Read the model definition and answer for the solid it produces. Units are mm, in the model's axes. Face numbers are marked on the shaded views. A direction names the side the tool comes from. Round coordinates to 2 decimals unless told otherwise and drop trailing zeros. Loops run counter-clockwise (first coordinate to the right, second up) from the corner with the lowest first, then second, coordinate; pieces in that order, holes last. Notation, with made-up numbers: (25.5, 24.25) -> (54.5, 24.25) arc R25 ccw to (54.5, 55.25) -> close; hole circle Ø10 at (-12.75, -29.5). An arc over 180 degrees is marked (long way). Put each result on its own line as item: value.
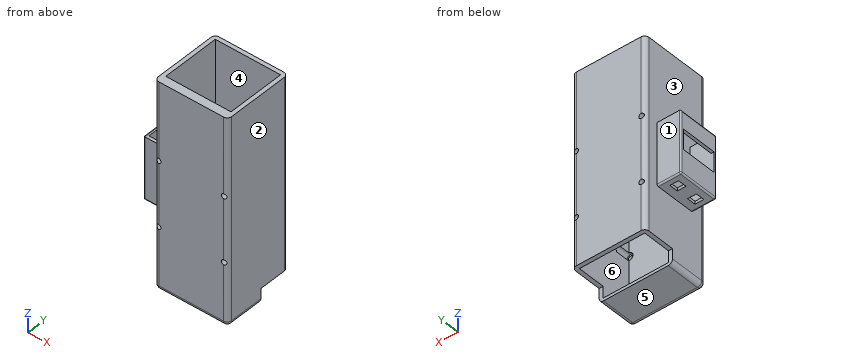
from build123d import *

# Parameters (mm, degrees)
SKETCH1_W           = 50.6
SKETCH1_H           = 45.6
SKETCH1_W_2         = 45
SKETCH1_H_2         = 40
BOSS_EXTRUDE1_DEPTH = 70
SKETCH2_W           = 50.6
SKETCH2_H           = 45.6
BOSS_EXTRUDE2_DEPTH = 2
SKETCH4_R           = 1.7
CUT_EXTRUDE1_DEPTH  = 71.5
SKETCH5_R           = 2.75
CUT_EXTRUDE2_DEPTH  = 12.5
SKETCH6_W           = 50.6
SKETCH6_H           = 4.293520681
BOSS_EXTRUDE3_DEPTH = 142
SKETCH7_R           = 1.7
CUT_EXTRUDE3_DEPTH  = 7.5
FILLET1_R           = 3
CUT_EXTRUDE4_DEPTH  = 22
BOSS_EXTRUDE4_DEPTH = 14.5
SKETCH10_W          = 43
SKETCH10_H          = 28.7
BOSS_EXTRUDE5_DEPTH = 2
SKETCH11_W          = 14
SKETCH11_H          = 24.7
CUT_EXTRUDE5_DEPTH  = 2
SKETCH12_W          = 6
SKETCH12_H          = 6
CUT_EXTRUDE6_DEPTH  = 2
FILLET2_R           = 1


with BuildPart() as part:
    # Sketch1 → Boss-Extrude1 (new, symmetric)
    with BuildSketch(Plane.XY):
        Rectangle(SKETCH1_W, SKETCH1_H)
        Rectangle(SKETCH1_W_2, SKETCH1_H_2, mode=Mode.SUBTRACT)
    extrude(amount=BOSS_EXTRUDE1_DEPTH, both=True)

    # Sketch2 → Boss-Extrude2 (add)
    with BuildSketch(Plane(origin=(0, 0, -70), x_dir=(-1, 0, 0), z_dir=(0, 0, -1))):
        Rectangle(SKETCH2_W, SKETCH2_H)
    extrude(amount=BOSS_EXTRUDE2_DEPTH)

    # Sketch4 → Cut-Extrude1 (cut)
    with BuildSketch(Plane(origin=(0, 22.8, 0), x_dir=(1, 0, 0), z_dir=(0, 1, 0))):
        with Locations(Location((-22.534370918, 28.890457594, 0), (0, 0, 270))):
            Circle(SKETCH4_R)
        with Locations(Location((22.465629082, 28.890457594, 0), (0, 0, 270))):
            Circle(SKETCH4_R)
        with Locations(Location((22.465629082, -16.109542406, 0), (0, 0, 270))):
            Circle(SKETCH4_R)
        with Locations(Location((-22.534370918, -16.109542406, 0), (0, 0, 270))):
            Circle(SKETCH4_R)
    extrude(amount=-CUT_EXTRUDE1_DEPTH, mode=Mode.SUBTRACT)

    # Sketch5 → Cut-Extrude2 (cut)
    with BuildSketch(Plane(origin=(0, -10, 0), x_dir=(1, 0, 0), z_dir=(0, 1, 0))):
        with Locations(Location((22.465629082, 28.890457594, 0), (0, 0, 270))):
            Circle(SKETCH5_R)
        with Locations(Location((22.465629082, -16.109542406, 0), (0, 0, 270))):
            Circle(SKETCH5_R)
        with Locations(Location((-22.534370918, 28.890457594, 0), (0, 0, 270))):
            Circle(SKETCH5_R)
        with Locations(Location((-22.534370918, -16.109542406, 0), (0, 0, 270))):
            Circle(SKETCH5_R)
    extrude(amount=-CUT_EXTRUDE2_DEPTH, mode=Mode.SUBTRACT)

    # Sketch6 → Boss-Extrude3 (add)
    with BuildSketch(Plane.XY.offset(70)):
        with Locations((0, -23.65323966)):
            Rectangle(SKETCH6_W, SKETCH6_H)
    extrude(amount=-BOSS_EXTRUDE3_DEPTH)

    # Sketch7 → Cut-Extrude3 (cut)
    with BuildSketch(Plane(origin=(0, -21.506479319, 0), x_dir=(1, 0, 0), z_dir=(0, 1, 0))):
        with Locations(Location((-22.534370918, 28.890457594, 0), (0, 0, 270))):
            Circle(SKETCH7_R)
        with Locations(Location((22.465629082, 28.890457594, 0), (0, 0, 270))):
            Circle(SKETCH7_R)
        with Locations(Location((22.465629082, -16.109542406, 0), (0, 0, 270))):
            Circle(SKETCH7_R)
        with Locations(Location((-22.534370918, -16.109542406, 0), (0, 0, 270))):
            Circle(SKETCH7_R)
    extrude(amount=-CUT_EXTRUDE3_DEPTH, mode=Mode.SUBTRACT)

    # Fillet1
    # the kernel refuses this fillet: 3 mm, written as the material it takes off along each edge
    with BuildSketch(Plane(origin=(-22.3, -22.8, -69), x_dir=(0, 0, -1), z_dir=(-1, 0, 0))) as fillet1_piece_1_section:
        Polygon((0, 0), (FILLET1_R, 0), (FILLET1_R, FILLET1_R), (0, FILLET1_R), align=None)
    fillet1_piece_1 = extrude(amount=FILLET1_R, mode=Mode.PRIVATE)
    fillet1_piece_1 = fillet1_piece_1 - Plane(origin=(-22.3, -22.8, -69), x_dir=(-2.085182079516792e-15, 0.7071067811865475, 0.7071067811865475), z_dir=(-1, 0, 0)) * Sphere(FILLET1_R, mode=Mode.PRIVATE)
    add(fillet1_piece_1, mode=Mode.SUBTRACT)
    with BuildSketch(Plane(origin=(22.3, -22.8, -69), x_dir=(0, -1, 0), z_dir=(0, 0, -1))) as fillet1_piece_2_section:
        Polygon((0, 0), (FILLET1_R, 0), (FILLET1_R, -FILLET1_R), (0, -FILLET1_R), align=None)
    fillet1_piece_2 = extrude(amount=FILLET1_R, mode=Mode.PRIVATE)
    fillet1_piece_2 = fillet1_piece_2 - Plane(origin=(22.3, -22.8, -69), x_dir=(-0.7071067811865486, 0.7071067811865464, 0), z_dir=(0, 0, -1)) * Sphere(FILLET1_R, mode=Mode.PRIVATE)
    add(fillet1_piece_2, mode=Mode.SUBTRACT)
    with BuildSketch(Plane(origin=(22.3, 19.8, -69), x_dir=(0, 0, -1), z_dir=(0, 1, 0))) as fillet1_piece_3_section:
        Polygon((0, 0), (FILLET1_R, 0), (FILLET1_R, -FILLET1_R), (0, -FILLET1_R), align=None)
    fillet1_piece_3 = extrude(amount=FILLET1_R, mode=Mode.PRIVATE)
    fillet1_piece_3 = fillet1_piece_3 - Plane(origin=(22.3, 19.8, -69), x_dir=(-0.7071067811865475, 0, 0.7071067811865475), z_dir=(0, 1, 0)) * Sphere(FILLET1_R, mode=Mode.PRIVATE)
    add(fillet1_piece_3, mode=Mode.SUBTRACT)
    with BuildSketch(Plane(origin=(-22.3, 19.8, -69), x_dir=(0, 1, 0), z_dir=(-1, 0, 0))) as fillet1_piece_4_section:
        Polygon((0, 0), (FILLET1_R, 0), (FILLET1_R, FILLET1_R), (0, FILLET1_R), align=None)
    fillet1_piece_4 = extrude(amount=FILLET1_R, mode=Mode.PRIVATE)
    fillet1_piece_4 = fillet1_piece_4 - Plane(origin=(-22.3, 19.8, -69), x_dir=(0, -0.7071067811865475, 0.7071067811865475), z_dir=(-1, 0, 0)) * Sphere(FILLET1_R, mode=Mode.PRIVATE)
    add(fillet1_piece_4, mode=Mode.SUBTRACT)
    with BuildSketch(Plane(origin=(-25.3, -25.8, 77.5), x_dir=(0, 1, 0), z_dir=(0, 0, -1)), Plane(origin=(25.3, -25.8, 77.5), x_dir=(-1, 0, 0), z_dir=(0, 0, -1))) as fillet1_piece_5:
        with BuildLine():
            CenterArc((FILLET1_R, FILLET1_R), FILLET1_R, 180, 90)
            Line((0, FILLET1_R), (0, 0))
            Line((0, 0), (FILLET1_R, 0))
        make_face()
    extrude(amount=146.5, mode=Mode.SUBTRACT)
    with BuildSketch(Plane(origin=(-22.3, -25.8, -72), x_dir=(0, 1, 0), z_dir=(1, 0, 0))) as fillet1_piece_6:
        with BuildLine():
            CenterArc((FILLET1_R, FILLET1_R), FILLET1_R, 180, 90)
            Line((0, FILLET1_R), (0, 0))
            Line((0, 0), (FILLET1_R, 0))
        make_face()
    extrude(amount=44.6, mode=Mode.SUBTRACT)
    with BuildSketch(Plane(origin=(25.3, 19.8, -72), x_dir=(-1, 0, 0), z_dir=(0, -1, 0)), Plane(origin=(-25.3, 19.8, -72), x_dir=(0, 0, 1), z_dir=(0, -1, 0))) as fillet1_piece_7:
        with BuildLine():
            CenterArc((FILLET1_R, -FILLET1_R), FILLET1_R, 90, 90)
            Line((0, -FILLET1_R), (0, 0))
            Line((0, 0), (FILLET1_R, 0))
        make_face()
    extrude(amount=42.6, mode=Mode.SUBTRACT)
    with BuildSketch(Plane(origin=(22.3, 22.8, -72), x_dir=(0, 0, 1), z_dir=(-1, 0, 0))) as fillet1_piece_8:
        with BuildLine():
            CenterArc((FILLET1_R, -FILLET1_R), FILLET1_R, 90, 90)
            Line((0, -FILLET1_R), (0, 0))
            Line((0, 0), (FILLET1_R, 0))
        make_face()
    extrude(amount=44.6, mode=Mode.SUBTRACT)
    with BuildSketch(Plane(origin=(25.3, 22.8, 77.5), x_dir=(-1, 0, 0), z_dir=(0, 0, -1)), Plane(origin=(-25.3, 22.8, 77.5), x_dir=(0, -1, 0), z_dir=(0, 0, -1))) as fillet1_piece_9:
        with BuildLine():
            CenterArc((FILLET1_R, -FILLET1_R), FILLET1_R, 90, 90)
            Line((0, -FILLET1_R), (0, 0))
            Line((0, 0), (FILLET1_R, 0))
        make_face()
    extrude(amount=146.5, mode=Mode.SUBTRACT)

    # Sketch8 → Cut-Extrude4 (cut)
    with BuildSketch(Plane.XZ.offset(-22.8)):
        Polygon((-25.3, -62), (25.3, -62), (25.3, -72), (25.3, -74.989483602), (-25.3, -74.989483602), align=None)
    extrude(amount=CUT_EXTRUDE4_DEPTH, mode=Mode.SUBTRACT)

    # Sketch9 → Boss-Extrude4 (add)
    with BuildSketch(Plane.ZY.offset(25.3)):
        Polygon((-25, 11.3), (16, 11.3), (16, 13.3), (-27, 13.3), (-27, -15.4), (16, -15.4), (16, -13.4), (-25, -13.4), align=None)
    extrude(amount=BOSS_EXTRUDE4_DEPTH)

    # Sketch10 → Boss-Extrude5 (add)
    with BuildSketch(Plane.ZY.offset(39.8)):
        with Locations((-5.5, -1.05)):
            Rectangle(SKETCH10_W, SKETCH10_H)
    extrude(amount=BOSS_EXTRUDE5_DEPTH)

    # Sketch11 → Cut-Extrude5 (cut)
    with BuildSketch(Plane.ZY.offset(41.8)):
        with Locations((-3, -1.05)):
            Rectangle(SKETCH11_W, SKETCH11_H)
    extrude(amount=-CUT_EXTRUDE5_DEPTH, mode=Mode.SUBTRACT)

    # Sketch12 → Cut-Extrude6 (cut)
    with BuildSketch(Plane(origin=(0, 0, -27), x_dir=(-1, 0, 0), z_dir=(0, 0, -1))):
        with Locations((33.55, 6.125)):
            Rectangle(SKETCH12_W, SKETCH12_H)
        with Locations((33.55, -8.225)):
            Rectangle(SKETCH12_W, SKETCH12_H)
    extrude(amount=-CUT_EXTRUDE6_DEPTH, mode=Mode.SUBTRACT)

    # Fillet2
    fillet2_edges = [part.edges().sort_by_distance(p)[0] for p in [
        (-33.55, 13.3, -27),
        (-33.55, -15.4, -27),
        (-41.8, -1.05, -27),
        (-41.8, -15.4, -5.5),
        (-41.8, -1.05, 16),
        (-41.8, 13.3, -5.5),
    ]]
    fillet(fillet2_edges, radius=FILLET2_R)


solid = part.part
Item 1: Which of the six approach directions +Z, -Z, +X, -X, +Y, -Y give full straight-line access (tool end or side, diameter ignored) to the marked faces 4, 5 and 6?
Derived:
face 4: +Z, -Z
face 5: -Z, +X, -X, +Y, -Y
face 6: +Z
Item 2: The part is cut by section A-A (z = 25.5). Determine the outline of the cut face in (x, y).
Derived:
outline: (-25.3, -22.8) arc R3 ccw to (-22.3, -25.8) -> (22.3, -25.8) arc R3 ccw to (25.3, -22.8) -> (25.3, 19.8) arc R3 ccw to (22.3, 22.8) -> (-22.3, 22.8) arc R3 ccw to (-25.3, 19.8) -> close; hole (-22.5, -20) -> (22.5, -20) -> (22.5, 20) -> (-22.5, 20) -> close
Item 3: Flat-ended cylindrical pins translate along their axes: pin 1 Ø0.8 at (x, z) = (-23.5, 17.5) entering from -Y; pin 2 Ø1 at (x, z) = (-32.5, -26) entering from +Y; pin 3 Ø1.4 at (x, z) = (24, 16) entering from -Y. Find the tip coordinate at first contact, or state that the pin passes through.
Derived:
pin 1: stops at y = -25.68
pin 2: stops at y = 13.3
pin 3: stops at y = -25.3
Item 4: The part is cut by section C-C (x = -7.5). Determine the outline of the cut face in (y, z), then the cut area to 3 significant figures.
Derived:
outline: (-25.8, -69) arc R3 ccw to (-22.8, -72) -> (0.8, -72) -> (0.8, -70) -> (-20, -70) -> (-20, 70) -> (-25.8, 70) -> close; (20, -62) -> (22.8, -62) -> (22.8, 70) -> (20, 70) -> close
area: 1,230 mm^2
Item 5: For a pull along Y with two mould halves and no side action, classify the marked faces 1, 2 and 3 as pulls with the +Y half, pulls with the -Y half, needs draft (parallel to the pull), parting line crosses it, or undercut.
Derived:
face 1: pulls with the +Y half
face 2: needs draft
face 3: undercut
Item 6: Find the intervals of material crossed by line 1 along X through (y, z) = (5, 6); line 2 along X through (y, z) = (-5.5, -47); line 3 along Y through (x, z) = (-8.5, 10), in increasing order.
Derived:
line 1: x = -41.8 to -39.8, -25.3 to -22.5, 22.5 to 25.3
line 2: x = -25.3 to -22.5, 22.5 to 25.3
line 3: y = -25.8 to -20, 20 to 22.8
